Work out the finished part from the listing and answer in its coordinate system (mm). A direction names the side the tool comes from. Round coordinates to 2 decimals unless told otherwise and drop trailing zeros. Loops run counter-clockwise (first coordinate to the right, second up) from the corner with the lowest first, then second, coordinate; pieces in that order, holes last.
Autodesk Inventor part; units mm, degrees
ref_plane "Work Plane4" through (42.5, 55, 0) normal (0, 0.3420201, -0.9396926) x (-1, 0, 0)
ref_plane "YZ Plane" through (0, 0, 0) normal (1, 0, 0) x (0, 1, 0)
ref_plane "XZ Plane" through (0, 0, 0) normal (0, 1, 0) x (-1, 0, 0)
sketch "Sketch1" plane through (0, 0, 0) normal (0, 0, 1) x (1, 0, 0)
  circle A0 centre (0, 0) radius 5
  circle A1 centre (65, 0) radius 5
  circle A2 centre (0, 0) radius 12.5
  circle A3 centre (65, 0) radius 12.5
  line L0 (22.5, 9.5) -> (42.5, 9.5)
  line L1 (42.5, 9.5) -> (42.5, -10.5)
  line L2 (42.5, -10.5) -> (22.5, -10.5)
  line L3 (22.5, -10.5) -> (22.5, 9.5)
  line L4 (0, 0) -> (65, 0) construction
  line L5 (32.5, 0) -> (32.5, 30) construction
  line L6 (27.5, 30) -> (37.5, 30)
  line L7 (12.5, 0) -> (12.5, 15)
  line L8 (52.5, 0) -> (52.5, 15)
  arc A4 (27.5, 30) -> (12.5, 15) centre (27.5, 15) ccw
  arc A5 (52.5, 15) -> (37.5, 30) centre (37.5, 15) ccw
  line L9 (-12.5, 0) -> (-12.5, 20)
  line L10 (77.5, 0) -> (77.5, 20)
  line L11 (22.5, 55) -> (42.5, 55)
  arc A6 (22.5, 55) -> (-12.5, 20) centre (22.5, 20) ccw
  arc A7 (77.5, 20) -> (42.5, 55) centre (42.5, 20) ccw
  point P0 (22.5, 30)
  point P1 (42.5, 30)
  dimension "d0" = 10
  dimension "d1" = 10
  dimension "d2" = 65
  dimension "d3" = 25
  dimension "d4" = 25
  dimension "d5" = 22.5
  dimension "d6" = 22.5
  dimension "d7" = 9.5
  dimension "d8" = 10.5
  dimension "d11" = 20
  dimension "d12" = 10
  dimension "d13" = 30
  dimension "d14" = 15
  dimension "d15" = 55
  dimension "d16" = 35
extrude "Extrusion1" add sketch "Sketch1" along normal blind 34 contours A0 | A1 | A2 | A2 L9 A6 L11 A7 L10 A3 L8 A5 L6 A4 L7 | A3
ref_plane "Work Plane4" through (42.5, 55, 0) normal (0, 0.3420201, -0.9396926) x (-1, 0, 0)
sketch "Sketch23" plane through (42.5, 55, 0) normal (0, 0.3420201, -0.9396926) x (-1, 0, 0)
  ellipse E0 centre (42.5, -40.0544) end of major axis (30, -40.0544) minor radius 11.7462 (30, -40.0544) -> (55, -40.0544) ccw
  line L0 (30, -40.0544) -> (30, -25.959)
  ellipse E1 centre (15, -25.959) end of major axis (30, -25.959) minor radius 14.0954 (30, -25.959) -> (15, -11.8636) ccw
  line L1 (15, -11.8636) -> (5, -11.8636)
  ellipse E2 centre (5, -25.959) end of major axis (20, -25.959) minor radius 14.0954 (5, -11.8636) -> (-10, -25.959) ccw
  line L2 (-10, -25.959) -> (-10, -40.0544)
  ellipse E3 centre (-22.5, -40.0544) end of major axis (-35, -40.0544) minor radius 11.7462 (-35, -40.0544) -> (-10, -40.0544) ccw
  line L3 (-35, -40.0544) -> (-35, -21.2606)
  ellipse E4 centre (0, -21.2606) end of major axis (-35, -21.2606) minor radius 32.8892 (0, 11.6287) -> (-35, -21.2606) ccw
  line L4 (0, 11.6287) -> (20, 11.6287)
  ellipse E5 centre (20, -21.2606) end of major axis (55, -21.2606) minor radius 32.8892 (55, -21.2606) -> (20, 11.6287) ccw
  line L5 (55, -21.2606) -> (55, -40.0544)
  ellipse E6 centre (42.5, -51.6831) end of major axis (30, -51.6831) minor radius 11.7462 (30, -51.6831) -> (55, -51.6831) ccw
  line L6 (55, -32.8892) -> (55, -51.6831)
  ellipse E7 centre (20, -32.8892) end of major axis (55, -32.8892) minor radius 32.8892 (55, -32.8892) -> (20, 0) ccw
  line L7 (0, 0) -> (20, 0)
  ellipse E8 centre (0, -32.8892) end of major axis (-35, -32.8892) minor radius 32.8892 (0, 0) -> (-35, -32.8892) ccw
  line L8 (-35, -51.6831) -> (-35, -32.8892)
  ellipse E9 centre (-22.5, -51.6831) end of major axis (-35, -51.6831) minor radius 11.7462 (-35, -51.6831) -> (-10, -51.6831) ccw
  line L9 (-10, -37.5877) -> (-10, -51.6831)
  ellipse E10 centre (5, -37.5877) end of major axis (20, -37.5877) minor radius 14.0954 (5, -23.4923) -> (-10, -37.5877) ccw
  line L10 (15, -23.4923) -> (5, -23.4923)
  ellipse E11 centre (15, -37.5877) end of major axis (30, -37.5877) minor radius 14.0954 (30, -37.5877) -> (15, -23.4923) ccw
  line L11 (30, -51.6831) -> (30, -37.5877)
  line L12 (0, 0) -> (20, 0)
  line L13 (10, 0) -> (10, -36)
  circle A0 centre (-22.5, -48.5) radius 5
  circle A1 centre (42.5, -48.5) radius 5
  circle A2 centre (-22.5, -48.5) radius 12.5
  circle A3 centre (42.5, -48.5) radius 12.5
  line L14 (-35, -36) -> (-10, -36)
  line L15 (-35, -36) -> (-35, -48.5)
  line L16 (-35, -51.6831) -> (-35, -40.0544)
  line L17 (-10, -36) -> (-10, -48.5)
  line L18 (-10, -51.6831) -> (-10, -40.0544)
  line L19 (30, -36) -> (55, -36)
  line L20 (30, -51.6831) -> (30, -40.0544)
  line L21 (30, -48.5) -> (30, -36)
  line L22 (55, -48.5) -> (55, -36)
  dimension "d108" = 36
  dimension "d110" = 10
  dimension "d111" = 10
  dimension "d112" = 12.5
  dimension "d113" = 12.5
  dimension "d114" = 25
  dimension "d115" = 25
extrude "Extrusion29" add sketch "Sketch23" against normal blind 49.285 contours L0 L19 A3 E0 | E0 A3 L11 | A3 E0 A1 | E0 A1 A3 | L19 L5 E0 A3 | A3 E0 L6 | L2 E3 A2 L14 | L9 A2 E3 | A2 E3 A0 | A2 E3 L3 L14 | A2 E3 A0 | A2 L8 E3
sketch "Sketch24" plane through (42.5, 55, 0) normal (0, 0.3420201, -0.9396926) x (-1, 0, 0)
  circle A0 centre (-22.5, -48.5) radius 5
  arc A1 (-35, -48.5) -> (-10, -48.5) centre (-22.5, -48.5) ccw
  line L0 (-10, -48.5) -> (-10, -36)
  line L1 (-10, -36) -> (-35, -36)
  line L2 (-35, -36) -> (-35, -48.5)
  circle A2 centre (42.5, -48.5) radius 5
  arc A3 (30, -48.5) -> (55, -48.5) centre (42.5, -48.5) ccw
  line L3 (55, -48.5) -> (55, -36)
  line L4 (30, -36) -> (55, -36)
  line L5 (30, -36) -> (30, -48.5)
  point P0 (42.5, -51.6831)
extrude "Extrusion30" cut sketch "Sketch24" against normal blind 13.103
sketch "Sketch25" plane through (77.5, 20, 34) normal (1, 0, 0) x (0, 0, -1)
  line L0 (1.5704, -20) -> (1.5704, -20)
  line L1 (1.5704, -20) -> (4.2752, -27.4316)
  line L2 (4.2752, -27.4316) -> (4.2752, -27.4316)
  line L3 (4.2752, -27.4316) -> (1.5704, -20)
  line L4 (-2.4671, -8.9071) -> (10.0523, -43.304)
  line L5 (10.0523, -43.304) -> (-2.0937, -47.7247)
  line L6 (-2.4671, -8.9071) -> (-14.6131, -13.3279)
  line L7 (-2.0937, -47.7247) -> (-14.6131, -13.3279)
  point P0 (34, -20)
extrude "Extrusion31" cut sketch "Sketch25" against normal blind 100
sketch "Sketch26" plane through (42.5, 50.5185, 12.3128) normal (0, 0.3420201, -0.9396926) x (-1, 0, 0)
  circle A0 centre (-22.5, -48.5) radius 5
  arc A1 (-35, -48.5) -> (-10, -48.5) centre (-22.5, -48.5) ccw
  line L0 (-10, -36.0002) -> (-10, -48.5)
  line L1 (-10, -36) -> (-10, -36.0002)
  line L2 (-35, -36) -> (-10, -36)
  line L3 (-35, -48.5) -> (-35, -36)
  circle A2 centre (42.5, -48.5) radius 5
  arc A3 (30, -48.5) -> (55, -48.5) centre (42.5, -48.5) ccw
  line L4 (55, -36) -> (55, -48.5)
  line L5 (30, -36) -> (55, -36)
  line L6 (30, -36.0002) -> (30, -36)
  line L7 (30, -48.5) -> (30, -36.0002)
  line L8 (-35, -36) -> (-43.7615, -36)
  line L9 (-43.7615, -36) -> (-43.7615, -67.4165)
  line L10 (-43.7615, -67.4165) -> (-2.78, -67.4165)
  line L11 (-2.78, -67.4165) -> (-2.78, -36)
  line L12 (-2.78, -36) -> (-10, -36)
  line L13 (30, -36.0002) -> (23.7348, -36)
  line L14 (23.7348, -36) -> (23.7338, -67.4165)
  line L15 (23.7338, -67.4165) -> (61.4136, -67.4165)
  line L16 (61.4136, -67.4165) -> (61.4136, -36.0012)
  line L17 (61.4136, -36.0012) -> (55, -36)
  point P0 (42.5, -51.6831)
extrude "Extrusion32" cut sketch "Sketch26" against normal blind 100 contours A0 | A1 L0 L12 L11 L10 L9 L8 L3 | A2 | A3 L4 L17 L16 L15 L14 L13 L7
sketch "Sketch27" plane through (22.5, 55, 0) normal (0, 1, 0) x (1, 0, 0)
  circle A0 centre (10, -17) radius 5
  line L0 (20, 0) -> (0, 0)
  line L1 (0, 0) -> (0, -34)
  line L2 (20, -34) -> (0, -34)
  line L3 (20, 0) -> (20, -34)
  point P0 (-22.5, 0)
  dimension "d124" = 10
  dimension "d125" = 20
  dimension "d126" = 34
  dimension "d127" = 10
  dimension "d128" = 17
extrude "Extrusion33" cut sketch "Sketch27" against normal blind 100 contours A0
sketch "Sketch28" plane through (42.5, 38.1435, 46.3128) normal (0, -0.3420201, 0.9396926) x (1, 0, 0)
  circle A0 centre (-42.5, -48.5) radius 5
  line L0 (-55, -48.5) -> (-55, -36)
  arc A1 (-55, -48.5) -> (-30, -48.5) centre (-42.5, -48.5) ccw
  line L1 (-30, -36) -> (-30, -48.5)
  line L2 (-55, -36) -> (-30, -36)
  circle A2 centre (22.5, -48.5) radius 5
  line L3 (35, -36) -> (35, -48.5)
  line L4 (35, -36) -> (10, -36)
  line L5 (10, -48.5) -> (10, -36)
  arc A3 (10, -48.5) -> (35, -48.5) centre (22.5, -48.5) ccw
  circle A4 centre (22.5, -48.5) radius 4.75
  circle A5 centre (22.5, -48.5) radius 5
  circle A6 centre (-42.5, -48.5) radius 5
  circle A7 centre (-42.5, -48.5) radius 4.75
  point P0 (-42.5, -51.6831)
  dimension "d131" = 9.5
  dimension "d132" = 9.5
extrude "Extrusion34" add sketch "Sketch28" against normal up to surface (36.182 mm away) contours A0 | A2
sketch "Sketch29" plane through (22.5, 55, 0) normal (0, 1, 0) x (1, 0, 0)
  circle A0 centre (10, -17) radius 5
  line L0 (20, 0) -> (0, 0)
  line L1 (0, 0) -> (0, -34)
  line L2 (20, -34) -> (0, -34)
  line L3 (20, 0) -> (20, -34)
  circle A1 centre (10, -17) radius 4.75
  point P0 (-22.5, 0)
  dimension "d135" = 9.5
extrude "Extrusion35" add sketch "Sketch29" against normal up to surface (25 mm away) contours A0
equation "\"d15\" = d13 + d3"
properties part number "MountB"
Item 1: Section A-A, the plane x = 32.5 is taken. Give the vertices of the cut face in (y, z).
Item 2: Each of these flat-tipped pins is pushed along its axis until it touches: P1, Ø12, axis at y = -7.5, z = 20, coming from the -X side; P2, Ø1, axis at y = 45.5, z = 3.5, coming from the +X side; P3, Ø11, axis at x = 32, z = 23.5, coming from the -Y side; P4, Ø1, axis at x = 57, y = -11.5, coming from the +Z side. Where does it stop, or does it pass through?
Item 3: Straight lines are drawn through the part: line 1 (Z direction, x = 32.5, y = 41); line 2 (X direction, y = 2, z = 2); line 3 (X direction, y = 7.5, z = 16). For each, find the intervals that lie inside material, in ascending order.
Item 4: Determine the mould class of faces 1 (the face through (32, 36, 0)), 2 (the face through (69.53, 0.01, 13.45)), 3 (the face through (-2.519, 44.475, 16.762)) for opening direction Y: pulls with the +Y half, pulls with the -Y half, needs draft (parallel to the pull), parting line crosses it, or undercut.
Item 5: Section D-D, the plane x = 20 is taken. Give the vertices of the cut face in (y, z), plus the area to 3 significant figures.
Item 6: For faces 4 (the face through (37.03, 42.68, 15.57)), 5 (the face through (47.99, 25.72, 16.76)), determine the directions among +Z, -Z, +X, -X, +Y, -Y from which every point of the face is accessible in a straight line to the end or side of a thin tool.
Item 7: Section B-B, the plane y = 11 is taken. Give the vertices of the cut face in (x, z).
Answer below:
1. outline: (30, 0) - (55, 0) - (55, 12.25) - (30, 12.25) - close; (30, 21.75) - (55, 21.75) - (55, 34) - (30, 34) - close
2. P1: stops at x = -12.5
2. P2: stops at x = 66.99
2. P3: stops at y = 29.97
2. P4: stops at z = 28.43
3. line 1: z = 0 to 12.25, 21.75 to 34
3. line 2: x = -12.48 to -4.71, 4.71 to 12.48, 52.52 to 60.29, 69.71 to 77.48
3. line 3: x = -12.5 to 12.5, 52.5 to 77.5
4. face 1: needs draft
4. face 2: undercut
4. face 3: pulls with the +Y half
5. outline: (27.99, 0) - (54.91, 0) - (54.91, 34) - (27.99, 34) - close
5. area: 915 mm2
6. face 4: +Y, -Y
6. face 5: +Z, -Z, -Y
7. outline: (-12.5, -2.07) - (12.5, -2.07) - (12.5, 34) - (-12.5, 34) - close; (52.5, -2.07) - (77.5, -2.07) - (77.5, 34) - (52.5, 34) - close
